Source: CAD feature listing. Evaluate the final solid. Frame: model axes, mm. Face numbers are marked on the shaded views. A direction names the side the tool comes from. Round coordinates to 2 decimals unless told otherwise and drop trailing zeros. Order: outer loops, then holes, each group sorted by start corner. A loop starts at its lowest first (then second) coordinate and runs counter-clockwise, first axis right, second up. Notation, with made-up numbers: (79.25, 15) - (97.25, 15) arc R28 ccw to (97.25, 46) - close; hole circle Ø11 at (-28.75, -32.75). An arc over 180 degrees is marked (long way). Use one line per item in the form item = value. Start each with the question number.
Q1. Set-up query: the marked faces 1, 2 and 3. Return all of +Z, -Z, +X, -X, +Y, -Y with unobstructed straight access to the full face (end or side cutting, diameter ignored); none if empty.
Q2. Cut plane A-A, the plane z = -12.5. Return the cut outline in (x, y), and give its area (3 significant figures).
Q3. Ray query, line 1 (Z direction, x = 20.5, y = 8.75); line 2 (Y direction, x = 6, z = -26.5); line 3 (Y direction, x = -2, z = -9.2). Return the intervals inside material, ascending. Write a range as [from, to].
Q4. Cut plane C-C, the plane y = 12.75. Return the cut outline in (x, z), and give its area (3 significant figures).
Q5. Cut plane B-B, the plane x = -1. Return the cut outline in (y, z), and give its area (3 significant figures).
Q6. Draft query along X for the marked faces 4, 5 and 6. Return one class per face: released by +X, released by -X, zero draft, split by the parting line, or undercut.
Q7. Pin query (flat end, axial travel): pin 1 Ø3 at (y, z) = (3.5, -5) entering from -X; pin 2 Ø2 at (x, y) = (7.5, 1.5) entering from +Z; pin 3 Ø5 at (x, y) = (11, 16.5) entering from +Z; pin 4 Ø1 at (x, y) = (-2, 4) entering from +Z. Return the tip coordinate at first contact, or that it passes through.
Q8. Cut plane D-D, the plane x = 12. Return the cut outline in (y, z).
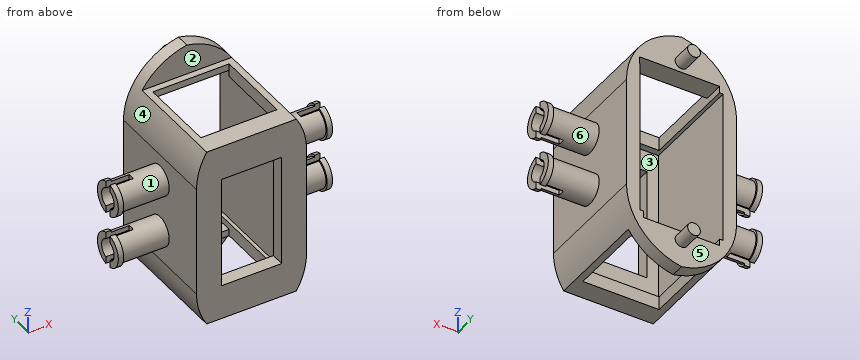
from build123d import *

# Parameters (mm, degrees)
SKETCH1_W           = 16.4
SKETCH1_H           = 27
BOSS_EXTRUDE1_DEPTH = 2
SKETCH5_W           = 16.4
SKETCH5_H           = 27
SKETCH5_W_2         = 12.4
SKETCH5_H_2         = 23
BOSS_EXTRUDE2_DEPTH = 15.5
SKETCH6_W           = 16.4
SKETCH6_H           = 2
BOSS_EXTRUDE3_DEPTH = 4.7
SKETCH7_W           = 16.4
SKETCH7_H           = 2
BOSS_EXTRUDE4_DEPTH = 4.7
SKETCH8_R           = 0.95
BOSS_EXTRUDE5_DEPTH = 3
FILLET1_R           = 10
SKETCH9_R           = 2.2
BOSS_EXTRUDE6_DEPTH = 6.96
BOSS_EXTRUDE7_START = 6.96
SKETCH10_R          = 2.2
BOSS_EXTRUDE7_DEPTH = 6.96
SKETCH11_W          = 11.35995283
SKETCH11_H          = 11.5
CUT_EXTRUDE1_DEPTH  = 45.277544069
SKETCH12_W          = 9
SKETCH12_H          = 16.693548388
CUT_EXTRUDE2_DEPTH  = 10
SKETCH14_W          = 11.35995283
SKETCH14_H          = 3
CUT_EXTRUDE5_DEPTH  = 1
SKETCH15_W          = 11.95995283
SKETCH15_H          = 3
CUT_EXTRUDE6_DEPTH  = 1
SKETCH16_R          = 2.5
BOSS_EXTRUDE8_DEPTH = 0.8
BOSS_EXTRUDE9_START = 0.8
SKETCH17_R          = 2.5
BOSS_EXTRUDE9_DEPTH = 0.8
SKETCH18_W          = 6.099763115
SKETCH18_H          = 1
CUT_EXTRUDE7_DEPTH  = 3.48
CUT_EXTRUDE8_DEPTH  = 3.48
SKETCH20_R          = 1.5
CUT_EXTRUDE9_DEPTH  = 7.76
CUT_EXTRUDE10_START = -7.76
SKETCH21_R          = 1.5
CUT_EXTRUDE10_DEPTH = 7.76


with BuildPart() as part:
    # Sketch1 → Boss-Extrude1 (new body)
    with BuildSketch(Plane(origin=(0, 0, 0), x_dir=(1, 0, 0), z_dir=(0, 1, 0))):
        with Locations((8.2, 13.5)):
            Rectangle(SKETCH1_W, SKETCH1_H)
    extrude(amount=BOSS_EXTRUDE1_DEPTH)

    # Sketch5 → Boss-Extrude2 (add)
    with BuildSketch(Plane(origin=(0, 2, 0), x_dir=(1, 0, 0), z_dir=(0, 1, 0))):
        with Locations((8.2, 13.5)):
            Rectangle(SKETCH5_W, SKETCH5_H)
        with Locations((8.2, 13.5)):
            Rectangle(SKETCH5_W_2, SKETCH5_H_2, mode=Mode.SUBTRACT)
    extrude(amount=BOSS_EXTRUDE2_DEPTH)

    # Sketch6 → Boss-Extrude3 (add)
    with BuildSketch(Plane(origin=(0, 0, -27), x_dir=(-1, 0, 0), z_dir=(0, 0, -1))):
        with Locations((-8.2, 16.5)):
            Rectangle(SKETCH6_W, SKETCH6_H)
    extrude(amount=BOSS_EXTRUDE3_DEPTH)

    # Sketch7 → Boss-Extrude4 (add)
    with BuildSketch(Plane.XY):
        with Locations((8.2, 16.5)):
            Rectangle(SKETCH7_W, SKETCH7_H)
    extrude(amount=BOSS_EXTRUDE4_DEPTH)

    # Sketch8 → Boss-Extrude5 (add)
    with BuildSketch(Plane(origin=(0, 17.5, 0), x_dir=(1, 0, 0), z_dir=(0, 1, 0))):
        with Locations(Location((8.2, 27.5, 0), (0, 0, 90))):
            Circle(SKETCH8_R)
        with Locations(Location((8.2, -0.5, 0), (0, 0, 90))):
            Circle(SKETCH8_R)
    extrude(amount=BOSS_EXTRUDE5_DEPTH)

    # Fillet1
    # the kernel refuses this fillet: 10 mm, written as the material it takes off along each edge
    with BuildSketch(Plane(origin=(16.4, -9.5, -31.7), x_dir=(0, 0, 1), z_dir=(0, 1, 0)), Plane(origin=(0, 42.5, -31.7), x_dir=(0, 0, 1), z_dir=(0, -1, 0)), Plane(origin=(16.4, 42.5, 4.7), x_dir=(0, 0, -1), z_dir=(0, -1, 0)), Plane(origin=(0, -9.5, 4.7), x_dir=(0, 0, -1), z_dir=(0, 1, 0))) as fillet1_piece_1:
        with BuildLine():
            CenterArc((FILLET1_R, -FILLET1_R), FILLET1_R, 90, 90)
            Line((0, -FILLET1_R), (0, 0))
            Line((0, 0), (FILLET1_R, 0))
        make_face()
    extrude(amount=52, mode=Mode.SUBTRACT)

    # Sketch9 → Boss-Extrude6 (add)
    with BuildSketch(Plane.ZY):
        with Locations(Location((-17.2, 8.75, 0), (0, 0, 180))):
            Circle(SKETCH9_R)
        with Locations(Location((-9.2, 8.75, 0), (0, 0, 180))):
            Circle(SKETCH9_R)
    extrude(amount=BOSS_EXTRUDE6_DEPTH)

    # Sketch10 → Boss-Extrude7 (add)
    with BuildSketch(Plane(origin=(16.4, 0, 0), x_dir=(0, 0, -1), z_dir=(1, 0, 0)).offset(BOSS_EXTRUDE7_START)):
        with Locations((9.2, 8.75)):
            Circle(SKETCH10_R)
        with Locations((17.2, 8.75)):
            Circle(SKETCH10_R)
    extrude(amount=-BOSS_EXTRUDE7_DEPTH)

    # Sketch11 → Cut-Extrude1 (cut, through all)
    with BuildSketch(Plane.XY):
        with Locations((8.2, 8.75)):
            Rectangle(SKETCH11_W, SKETCH11_H)
    extrude(amount=-CUT_EXTRUDE1_DEPTH, mode=Mode.SUBTRACT)

    # Sketch12 → Cut-Extrude2 (cut)
    with BuildSketch(Plane(origin=(0, 2, 0), x_dir=(1, 0, 0), z_dir=(0, 1, 0))):
        with Locations((8.2, 13.5)):
            Rectangle(SKETCH12_W, SKETCH12_H)
    extrude(amount=-CUT_EXTRUDE2_DEPTH, mode=Mode.SUBTRACT)

    # Sketch14 → Cut-Extrude5 (cut)
    with BuildSketch(Plane.XY.offset(-25)):
        with Locations((8.2, 16)):
            Rectangle(SKETCH14_W, SKETCH14_H)
    extrude(amount=-CUT_EXTRUDE5_DEPTH, mode=Mode.SUBTRACT)

    # Sketch15 → Cut-Extrude6 (cut)
    with BuildSketch(Plane(origin=(0, 0, -2), x_dir=(-1, 0, 0), z_dir=(0, 0, -1))):
        with Locations((-8.5, 16)):
            Rectangle(SKETCH15_W, SKETCH15_H)
    extrude(amount=-CUT_EXTRUDE6_DEPTH, mode=Mode.SUBTRACT)

    # Sketch16 → Boss-Extrude8 (add)
    with BuildSketch(Plane(origin=(23.36, 0, 0), x_dir=(0, 0, -1), z_dir=(1, 0, 0))):
        with Locations((9.2, 8.75)):
            Circle(SKETCH16_R)
        with Locations((17.2, 8.75)):
            Circle(SKETCH16_R)
    extrude(amount=BOSS_EXTRUDE8_DEPTH)

    # Sketch17 → Boss-Extrude9 (add)
    with BuildSketch(Plane.ZY.offset(6.96).offset(BOSS_EXTRUDE9_START)):
        with Locations(Location((-9.2, 8.75, 0), (0, 0, 180))):
            Circle(SKETCH17_R)
        with Locations(Location((-17.2, 8.75, 0), (0, 0, 180))):
            Circle(SKETCH17_R)
    extrude(amount=-BOSS_EXTRUDE9_DEPTH)

    # Sketch18 → Cut-Extrude7 (cut)
    with BuildSketch(Plane.ZY.offset(7.76)):
        with Locations((-17.37045616, 8.75)):
            Rectangle(SKETCH18_W, SKETCH18_H)
        Polygon((-6.209519779, 8.75), (-6.209519779, 8.25), (-12.153333116, 8.25), (-12.153333116, 9.25), (-6.209519779, 9.25), align=None)
    extrude(amount=-CUT_EXTRUDE7_DEPTH, mode=Mode.SUBTRACT)

    # Sketch19 → Cut-Extrude8 (cut)
    with BuildSketch(Plane(origin=(24.16, 0, 0), x_dir=(0, 0, -1), z_dir=(1, 0, 0))):
        Polygon((6.297180826, 8.75), (6.297180826, 9.25), (20.308323275, 9.25), (20.308323275, 8.25), (6.297180826, 8.25), align=None)
    extrude(amount=-CUT_EXTRUDE8_DEPTH, mode=Mode.SUBTRACT)

    # Sketch20 → Cut-Extrude9 (cut)
    with BuildSketch(Plane(origin=(24.16, 0, 0), x_dir=(0, 0, -1), z_dir=(1, 0, 0))):
        with Locations((9.2, 8.75)):
            Circle(SKETCH20_R)
        with Locations((17.2, 8.75)):
            Circle(SKETCH20_R)
    extrude(amount=-CUT_EXTRUDE9_DEPTH, mode=Mode.SUBTRACT)

    # Sketch21 → Cut-Extrude10 (cut)
    with BuildSketch(Plane.ZY.offset(7.76).offset(CUT_EXTRUDE10_START)):
        with Locations(Location((-9.2, 8.75, 0), (0, 0, 180))):
            Circle(SKETCH21_R)
        with Locations(Location((-17.2, 8.75, 0), (0, 0, 180))):
            Circle(SKETCH21_R)
    extrude(amount=CUT_EXTRUDE10_DEPTH, mode=Mode.SUBTRACT)


solid = part.part
Completed:
q1.face_1 = none
q1.face_2 = +Z, +X, -X, -Y
q1.face_3 = +Y
q2.outline = (0, 0) - (3.7, 0) - (3.7, 2) - (2, 2) - (2, 17.5) - (0, 17.5) - close; (12.7, 0) - (16.4, 0) - (16.4, 17.5) - (14.4, 17.5) - (14.4, 2) - (12.7, 2) - close
q2.area = 76.8 mm2
q3.line_1 = [-19.4, -18.7], [-15.7, -15], [-11.4, -10.7], [-7.7, -7]
q3.line_2 = [0, 3], [14.5, 17.5]
q3.line_3 = [6.55, 7.25], [10.25, 10.95]
q4.outline = (0, -21.7) arc R10 ccw to (1.52, -27) - (2.52, -27) - (2.52, -25) - (2, -25) - (2, -2) - (2.52, -2) - (2.52, 0) - (1.52, 0) arc R10 ccw to (0, -5.3) - close; (13.88, -27) - (14.88, -27) arc R10 ccw to (16.4, -21.7) - (16.4, -5.3) arc R10 ccw to (14.88, 0) - (13.88, 0) - (13.88, -2) - (14.4, -2) - (14.4, -25) - (13.88, -25) - close
q4.area = 102 mm2
q5.outline = circle Ø4.4 at (8.75, -17.2); circle Ø4.4 at (8.75, -9.2); hole circle Ø3 at (8.75, -17.2); hole circle Ø3 at (8.75, -9.2)
q5.area = 16.3 mm2
q6.face_4 = released by -X
q6.face_5 = zero draft
q6.face_6 = undercut
q7.pin_1 = 0
q7.pin_2 = 0
q7.pin_3 = 4.48
q7.pin_4 = through
q8.outline = (0, -27) - (3, -27) - (3, -25) - (2, -25) - (2, -21.85) - (0, -21.85) - close; (0, -5.15) - (2, -5.15) - (2, -2) - (3, -2) - (3, 0) - (0, 0) - close; (14.5, -27) - (15.5, -27) - (15.5, -29.98) - (17.5, -29.98) - (17.5, -26) - (14.5, -26) - close; (14.5, -1) - (17.5, -1) - (17.5, 2.98) - (15.5, 2.98) - (15.5, 0) - (14.5, 0) - close
